```python
from build123d import *

# Parameters (mm, degrees)
F0_R     = 10
F1_DEPTH = 25
F2_DEPTH = 50
F3_SIZE  = 5


with BuildPart() as f1:
    # F0 (on Front) → F1 (new body)
    with BuildSketch(Plane.XZ):
        with BuildLine():
            ThreePointArc((2.083333, 24.913043), (18.399502, 16.92508), (25, 0))
            ThreePointArc((25, 0), (18.399502, -16.92508), (2.083333, -24.913043))
            Line((2.083333, -24.913043), (91.458333, -17.43913))
            ThreePointArc((91.458333, -17.43913), (72.5, 0), (91.458333, 17.43913))
            Line((91.458333, 17.43913), (2.083333, 24.913043))
        make_face()
        with BuildLine():
            ThreePointArc((107.5, 0), (102.879651, 11.847556), (91.458333, 17.43913))
            ThreePointArc((91.458333, 17.43913), (72.5, 0), (91.458333, -17.43913))
            ThreePointArc((91.458333, -17.43913), (102.879651, -11.847556), (107.5, 0))
        make_face()
        with Locations((90, 0)):
            Circle(F0_R, mode=Mode.SUBTRACT)
        with BuildLine():
            ThreePointArc((2.083333, -24.913043), (18.399502, -16.92508), (25, 0))
            ThreePointArc((25, 0), (18.399502, 16.92508), (2.083333, 24.913043))
            ThreePointArc((2.083333, 24.913043), (-25, 0), (2.083333, -24.913043))
        make_face()
        Circle(F0_R, mode=Mode.SUBTRACT)
    extrude(amount=F1_DEPTH)

    # F0 (on Front) → F2 (join)
    with BuildSketch(Plane.XZ):
        with BuildLine():
            ThreePointArc((2.083333, -24.913043), (18.399502, -16.92508), (25, 0))
            ThreePointArc((25, 0), (18.399502, 16.92508), (2.083333, 24.913043))
            ThreePointArc((2.083333, 24.913043), (-25, 0), (2.083333, -24.913043))
        make_face()
        Circle(F0_R, mode=Mode.SUBTRACT)
    extrude(amount=F2_DEPTH)

    # F3
    f3_edges = [f1.edges().sort_by_distance(p)[0] for p in [
        (-2.083333, -50, 24.913043),
        (-10, -50, 0),
        (80, -25, 0),
    ]]
    chamfer(f3_edges, length=F3_SIZE)


solid = f1.part
```
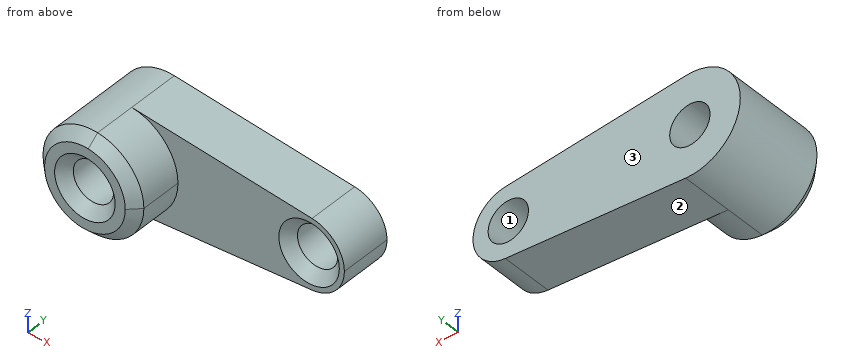
Source: CAD feature listing. Evaluate the final solid. Frame: model axes, mm. Face numbers are marked on the shaded views. Coordinates: 2 decimals unless noted, no trailing zeros. Order: outer loops, then holes, each group sorted by start corner. A loop starts at its lowest first (then second) coordinate and runs counter-clockwise, first axis right, second up. Notation, with made-up numbers: M 33.25,-16.75 L 51.25,-16.75 A15 ccw 51.25,9.25 Z; hole C 17.25,70.25 d7. An arc over 180 degrees is marked long. Write each question's results on one line, items separated by ' | '. Start each with the question number.
1) Section query B-B (y = -14). Return the cut outline in (x, z).
2) Line query: line 1 (Z direction, x = 0, y = -14); line 2 (X direction, y = -9.5, z = 6.5); line 3 (Y direction, x = 59, z = 4.5). Output: solid intervals per line, ascending. Write a range as from..to.
3) Draft query along X for the marked faces 1, 2 and 3. Return one class per face: released by +X, released by -X, zero draft, split by the parting line, or undercut.
4) Section query C-C (y = -30). Return the cut outline in (x, z), plus the area to 3 significant figures.
5) Section query D-D (z = 4). Give the number of separate pieces and of enclosed holes in the cut face, plus the area to 3 significant figures.
6) Contact query for flat-ended pins moving along their axis: pin 1 Ø6 at (x, y) = (7.5, -33.5) entering from -Z; pin 2 Ø6 at (x, y) = (72, -17.5) entering from +Z; pin 3 Ø2 at (y, z) = (-35, -1) entering from -X; pin 4 Ø16 at (x, z) = (90, 0) entering from -Y. Output: stop coordinate, or through.
7) Section query A-A (x = 0). Return the cut outline in (y, z), plus the area to 3 significant figures.
Answers:
1) outline: M 2.08,-24.91 L 91.46,-17.44 A17.5 ccw 91.46,17.44 L 2.08,24.91 A25 ccw long Z; hole C 0,0 d20; hole C 90,0 d20
2) line 1: z = -25..-10, 10..25 | line 2: x = -24.14..-7.6, 7.6..82.4, 97.6..106.25 | line 3: y = -25..0
3) face 1: undercut | face 2: released by +X | face 3: zero draft
4) outline: M 2.08,-24.91 A25 ccw 25,0 A25 ccw 2.08,24.91 A25 ccw long Z; hole C 0,0 d20 | area: 1,650 mm^2
5) separate pieces: 3 | enclosed holes: 0 | area: 3,070 mm^2
6) pin 1: stops at z = -24.59 | pin 2: stops at z = 19.32 | pin 3: stops at x = -25 | pin 4: passes through
7) outline: M -50,-20 L -45,-25 L 0,-25 L 0,-10 L -45,-10 L -50,-15 Z; M -50,15 L -45,10 L 0,10 L 0,25 L -45,25 L -50,20 Z | area: 1,450 mm^2
